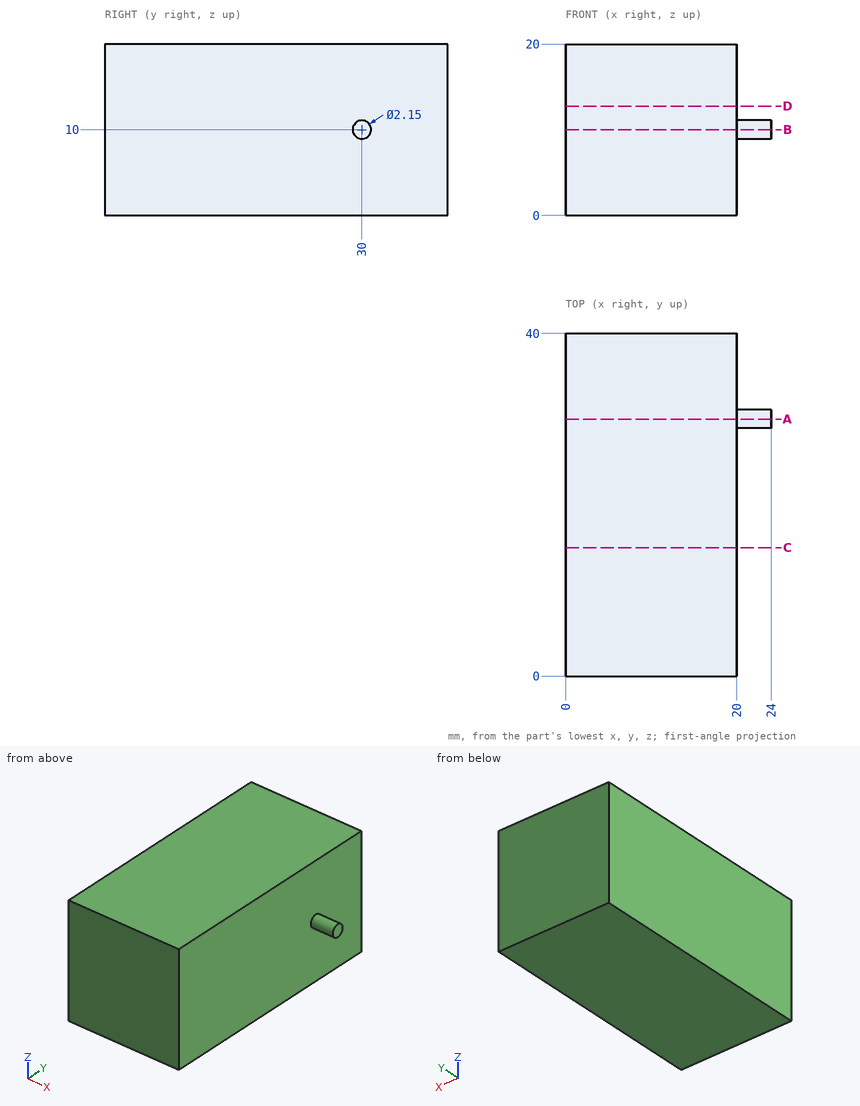
Part print with two shaded views. Sizes in mm from the minimum x, y, z corner. Give positions to 0.01 mm unless a question says otherwise; leave off trailing zeros. Loops run counter-clockwise (first coordinate to the right, second up) from the corner with the lowest first, then second, coordinate; pieces in that order, holes last. Notation, with made-up numbers: (18, -24) -> (25, -24) arc R23 cw to (25, 15) -> close; hole circle Ø11 at (-18.75, 28). An arc over 180 degrees is marked (long way). One line per question, with ' | ' between items.
Q1. Cut at A-A, the plane y = 30. Write the cut outline in (x, z) (1 decimal), plus the area to 3 significant figures.
Filled sheet:
outline: (0, 0) -> (20, 0) -> (20, 8.9) -> (24, 8.9) -> (24, 11.1) -> (20, 11.1) -> (20, 20) -> (0, 20) -> close | area: 409 mm²
Q2. Drill centre line: line 1 along X through (y, z) = (34.5, 2.75). Where is it in solid material? Low to high. Write a range as [from, to].
Filled sheet:
line 1: x = [0, 20]
Q3. Cut at D-D, the plane z = 12.75. Write the cut outline in (x, y), plus the area to 3 significant figures.
Filled sheet:
outline: (0, 0) -> (20, 0) -> (20, 40) -> (0, 40) -> close | area: 800 mm²
Q4. Cut at C-C, the plane y = 15. Write the cut outline in (x, z).
Filled sheet:
outline: (0, 0) -> (20, 0) -> (20, 20) -> (0, 20) -> close
Q5. Drop flat-ended pins along their axis: pin 1 (5 mm diameter, centred on y = 8.5, z = 15.5, fed in from +X); pin 2 (4 mm diameter, centred on y = 8.5, z = 18, fed in from -X). Give the stop position or say it passes through.
Filled sheet:
pin 1: stops at x = 20 | pin 2: stops at x = 0
Q6. Cut at B-B, the plane z = 10. Write the cut outline in (x, y) (1 decimal).
Filled sheet:
outline: (0, 0) -> (20, 0) -> (20, 28.9) -> (24, 28.9) -> (24, 31.1) -> (20, 31.1) -> (20, 40) -> (0, 40) -> close
